The model under review builds one solid part; all positions refer to its coordinate system, in mm. A direction names the side the tool comes from. Round coordinates to 2 decimals unless told otherwise and drop trailing zeros. Loops run counter-clockwise (first coordinate to the right, second up) from the corner with the lowest first, then second, coordinate; pieces in that order, holes last. Notation, with made-up numbers: (19, 82) -> (66, 82) arc R28 cw to (66, 100) -> close; hole circle Ø3 at (-10.75, 58.5). An arc over 180 degrees is marked (long way). Return JSON: item names as keys, results as strings. Group by question number.
```python
from build123d import *

# Parameters (mm, degrees)
F0_R     = 8.5
F0_R_2   = 1
F1_DEPTH = 3
F2_R     = 9.05
F3_DEPTH = 2.5
F4_W     = 1.5
F4_H     = 1.5
F5_DEPTH = 3
F6_SIZE  = 0.5


with BuildPart() as f1:
    # F0 (on Top) → F1 (new body)
    with BuildSketch(Plane.XY):
        with BuildLine():
            Line((20.3929555267, 13.1650441562), (-30.6070444733, 13.1650441562))
            Line((-30.6070444733, 13.1650441562), (-30.6070444733, -7.7349558438))
            Line((-30.6070444733, -7.7349558438), (-9.3570444733, -7.7349558438))
            Line((-9.3570444733, -7.7349558438), (-9.3570444733, -6.2349558438))
            Line((-9.3570444733, -6.2349558438), (-7.8570444733, -6.2349558438))
            Line((-7.8570444733, -6.2349558438), (-7.8570444733, -7.7349558438))
            Line((-7.8570444733, -7.7349558438), (9.6429555267, -7.7349558438))
            Line((9.6429555267, -7.7349558438), (9.6429555267, -6.2349558438))
            Line((9.6429555267, -6.2349558438), (11.1429555267, -6.2349558438))
            Line((11.1429555267, -6.2349558438), (11.1429555267, -7.7349558438))
            Line((11.1429555267, -7.7349558438), (20.3929555267, -7.7349558438))
            Line((20.3929555267, -7.7349558438), (20.3929555267, -4.2849558438))
            ThreePointArc((20.3929555267, -4.2849558438), (21.4180817926, -1.8100821097), (23.8929555267, -0.7849558438))
            Line((23.8929555267, -0.7849558438), (32.3929555267, -0.7849558438))
            Line((32.3929555267, -0.7849558438), (32.3929555267, 6.2150441562))
            Line((32.3929555267, 6.2150441562), (23.8929555267, 6.2150441562))
            ThreePointArc((23.8929555267, 6.2150441562), (21.4180817926, 7.240170422), (20.3929555267, 9.7150441562))
            Line((20.3929555267, 9.7150441562), (20.3929555267, 13.1650441562))
        make_face()
        with Locations((-0.8570444733, 2.7150441562)):
            Circle(F0_R, mode=Mode.SUBTRACT)
        with Locations((-19.8570444733, 2.7150441562)):
            Circle(F0_R, mode=Mode.SUBTRACT)
        with Locations((-12.3570444733, 11.1650441562)):
            Circle(F0_R_2, mode=Mode.SUBTRACT)
    extrude(amount=F1_DEPTH)

    # F2 (on face) → F3 (cut)
    with BuildSketch(Plane.XY.offset(3)):
        with Locations((-19.8570444733, 2.7150441562)):
            Circle(F2_R)
    extrude(amount=-F3_DEPTH, mode=Mode.SUBTRACT)

    # F4 (on face) → F5 (cut)
    with BuildSketch(Plane.XY.offset(3)):
        with Locations((28.1429555267, -0.0349558438)):
            Rectangle(F4_W, F4_H)
        with Locations((28.1429555267, 5.4650441562)):
            Rectangle(F4_W, F4_H)
    extrude(amount=-F5_DEPTH, mode=Mode.SUBTRACT)

    # F6
    f6_edges = [f1.edges().sort_by_distance(p)[0] for p in [
        (27.392956, -0.784956, 1.5),
        (28.892956, -0.784956, 1.5),
        (28.892956, 6.215044, 1.5),
        (27.392956, 6.215044, 1.5),
    ]]
    chamfer(f6_edges, length=F6_SIZE)


solid = f1.part
```
1. Draft analysis for pull direction X (two halves, no side actions). For faces 1 (the face through (32.393, 3, 1)), 2 (the face through (28, 0.715, 2)), 3 (the face through (25, 6.215, 1)), 4 (the face through (-11.75, 5.27, 0.25)), state which applies: pulls with the +X half, pulls with the -X half, needs draft (parallel to the pull), parting line crosses it, or undercut.
2. We need section A-A, the plane y = -1.5. Write out the cut boundary in (x, z), then the cut area to 3 significant figures.
3. For P1, Ø0.8, axis at x = 10.5, z = 1.5, coming from the -Y side; P2, Ø1.2, axis at y = -6.5, z = 1.5, coming from the +X side; P3, Ø1.2, axis at x = -12.36, y = 11.17, coming from the -Z side; P4, Ø1.5, axis at x = 30.5, z = 2, coming from the +Y side, all flat-tipped, find the tip position at first contact; note any pin that passes through.
4. Tool access review of faces 5 (the face through (20.393, 11, 1)), 6 (the face through (-30.607, 3, 1)), 7 (the face through (-9.357, -7, 1)), 8 (the face through (27.393, 5, 2)): name each direction out of +Z, -Z, +X, -X, +Y, -Y from which nothing blocks a thin tool from reaching the whole face with its end or side.
5. We need section B-B, the plane x = -2. Write out the cut boundary in (y, z).
6. Wall thickness on line 1 (X direction, y = 9, z = 1.7); line 2 (X direction, y = 8.75, z = 2.15); line 3 (X direction, y = 5.75, z = 0.3): over which ranges is each line inside the solid? List them lowest first.
7. We need section D-D, the plane y = 1.5. Write out the cut boundary in (x, z).
8. We need section C-C, the plane z = 2.2. Give the number of separate pieces and of enclosed holes in the cut face, then the cut area to 3 significant figures.
Check sheet entries:
{
 "1": {"face 1": "pulls with the +X half", "face 2": "undercut", "face 3": "needs draft", "face 4": "undercut"},
 "2": {"outline": "(-30.61, 0) -> (-27.24, 0) -> (-27.24, 0.5) -> (-27.87, 0.5) -> (-27.87, 3) -> (-30.61, 3) -> close; (-12.48, 0) -> (-8.24, 0) -> (-8.24, 3) -> (-11.85, 3) -> (-11.85, 0.5) -> (-12.48, 0.5) -> close; (6.52, 0) -> (21.77, 0) -> (21.77, 3) -> (6.52, 3) -> close", "area": "65.4 mm²"},
 "3": {"P1": "stops at y = -6.23", "P2": "stops at x = 20.39", "P3": "passes through", "P4": "stops at y = 6.22"},
 "4": {"face 5": "+Z, -Z, +X, +Y", "face 6": "+Z, -Z, -X, +Y, -Y", "face 7": "+Z, -Z, -Y", "face 8": "+Z, -Z, +Y"},
 "5": {"outline": "(-7.73, 0) -> (-5.71, 0) -> (-5.71, 3) -> (-7.73, 3) -> close; (11.14, 0) -> (13.17, 0) -> (13.17, 3) -> (11.14, 3) -> close"},
 "6": {"line 1": "x = -30.61 to -26.37, -13.35 to -6.58, 4.87 to 20.47", "line 2": "x = -30.61 to -26.6, -13.11 to -6.84, 5.13 to 20.53", "line 3": "x = -30.61 to -27.8, -11.92 to -8.8, 7.08 to 27.36, 28.93 to 32.39"},
 "7": {"outline": "(-30.61, 0) -> (-28.27, 0) -> (-28.27, 0.5) -> (-28.83, 0.5) -> (-28.83, 3) -> (-30.61, 3) -> close; (-11.44, 0) -> (-9.27, 0) -> (-9.27, 3) -> (-10.89, 3) -> (-10.89, 0.5) -> (-11.44, 0.5) -> close; (7.56, 0) -> (32.39, 0) -> (32.39, 3) -> (7.56, 3) -> close"},
 "8": {"separate pieces": "1", "enclosed holes": "3", "area": "658 mm²"}
}
